Check sheet for the modelled part. Datum: model origin and axes. Units: mm. Face numbers are marked on the shaded views. A direction names the side the tool comes from. Coordinates: 2 decimals unless noted, no trailing zeros. Loops run counter-clockwise (first coordinate to the right, second up) from the corner with the lowest first, then second, coordinate; pieces in that order, holes last. Notation, with made-up numbers: M 71,42.5 L 109,42.5 A20 cw 109,62.5 Z; hole C 22.25,-23 d2. An arc over 180 degrees is marked long. Write each question's results on one line, items separated by ' | '. Start each with the question number.
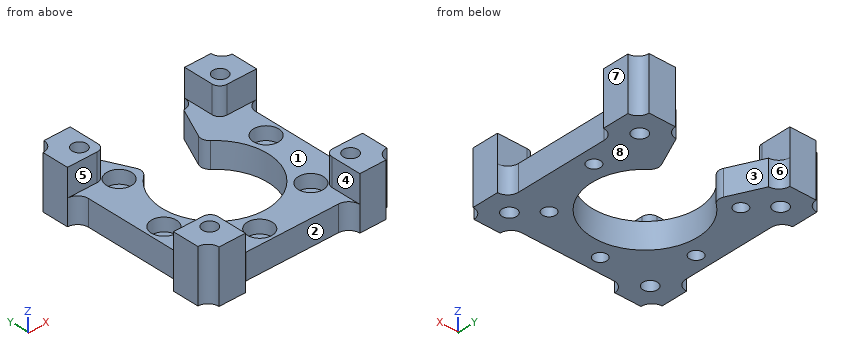
from build123d import *

# Parameters (mm, degrees)
SKETCH_R     = 1.5
SKETCH_R_2   = 1.65
PAD_DEPTH    = 5.8
SKETCH001_R  = 1.65
PAD001_DEPTH = 6.2
SKETCH002_R  = 2.85
POCKET_DEPTH = 3


with BuildPart() as part:
    # Sketch → Pad (new body)
    with BuildSketch(Plane.XY):
        with BuildLine():
            ThreePointArc((-21.5, 19), (-19.732233, 19.732233), (-19, 21.5))
            Line((-19, 21.5), (-13, 21.5))
            ThreePointArc((-13, 21.5), (-12.267767, 19.732233), (-10.500001, 19))
            Line((-10.500001, 19), (-7.065457, 11.675563))
            ThreePointArc((-7.608223, 9.279814), (-6.925691, 10.384542), (-7.065457, 11.675563))
            ThreePointArc((-7.608223, 9.279814), (0, -12), (7.608223, 9.279814))
            ThreePointArc((7.065457, 11.675563), (6.925691, 10.384541), (7.608223, 9.279814))
            Line((10.500001, 19), (7.065457, 11.675563))
            ThreePointArc((10.500001, 19), (12.267767, 19.732233), (13, 21.5))
            Line((19, 21.5), (13, 21.5))
            ThreePointArc((19, 21.5), (19.732233, 19.732233), (21.5, 19))
            Line((21.5, 19), (21.5, 13))
            ThreePointArc((21.5, 13), (19.732233, 12.267767), (19, 10.500001))
            Line((19, 10.500001), (19, -10.500001))
            ThreePointArc((19, -10.500001), (19.732233, -12.267767), (21.5, -13))
            Line((21.5, -19), (21.5, -13))
            ThreePointArc((21.5, -19), (19.732233, -19.732233), (19, -21.5))
            Line((19, -21.5), (13, -21.5))
            ThreePointArc((13, -21.5), (12.267767, -19.732233), (10.500001, -19))
            Line((10.500001, -19), (-10.500001, -19))
            ThreePointArc((-10.500001, -19), (-12.267767, -19.732233), (-13, -21.5))
            Line((-19, -21.5), (-13, -21.5))
            ThreePointArc((-19, -21.5), (-19.732233, -19.732233), (-21.5, -19))
            Line((-21.5, -19), (-21.5, -13))
            ThreePointArc((-21.5, -13), (-19.732233, -12.267767), (-19, -10.500001))
            Line((-19, 10.500001), (-19, -10.500001))
            ThreePointArc((-19, 10.500001), (-19.732233, 12.267767), (-21.5, 13))
            Line((-21.5, 19), (-21.5, 13))
        make_face()
        with Locations((-11.313708, 11.313708)):
            Circle(SKETCH_R, mode=Mode.SUBTRACT)
        with Locations((-15.454813, -4.141105)):
            Circle(SKETCH_R, mode=Mode.SUBTRACT)
        with Locations((-4.141105, -15.454813)):
            Circle(SKETCH_R, mode=Mode.SUBTRACT)
        with Locations((11.313708, -11.313708)):
            Circle(SKETCH_R, mode=Mode.SUBTRACT)
        with Locations((15.454813, 4.141105)):
            Circle(SKETCH_R, mode=Mode.SUBTRACT)
        with Locations((-16, 16)):
            Circle(SKETCH_R_2, mode=Mode.SUBTRACT)
        with Locations((16, 16)):
            Circle(SKETCH_R_2, mode=Mode.SUBTRACT)
        with Locations((16, -16)):
            Circle(SKETCH_R_2, mode=Mode.SUBTRACT)
        with Locations((-16, -16)):
            Circle(SKETCH_R_2, mode=Mode.SUBTRACT)
    extrude(amount=PAD_DEPTH)

    # Sketch001 (on Face39 of Pad) → Pad001 (join)
    with BuildSketch(Plane.XY.offset(5.8)):
        with BuildLine():
            ThreePointArc((-21.5, 19), (-19.732233, 19.732233), (-19, 21.5))
            Line((-19, 21.5), (-13, 21.5))
            Line((-13, 21.5), (-13, 14.726703))
            ThreePointArc((-14.726703, 13), (-13.50574, 13.50574), (-13, 14.726703))
            Line((-21.5, 13), (-14.726703, 13))
            Line((-21.5, 19), (-21.5, 13))
        make_face()
        with Locations((-16, 16)):
            Circle(SKETCH001_R, mode=Mode.SUBTRACT)
        with BuildLine():
            ThreePointArc((-19, -21.5), (-19.732233, -19.732233), (-21.5, -19))
            Line((-21.5, -19), (-21.5, -13))
            Line((-21.5, -13), (-14.726703, -13))
            ThreePointArc((-13, -14.726703), (-13.50574, -13.50574), (-14.726703, -13))
            Line((-13, -21.5), (-13, -14.726703))
            Line((-19, -21.5), (-13, -21.5))
        make_face()
        with Locations((-16, -16)):
            Circle(SKETCH001_R, mode=Mode.SUBTRACT)
        with BuildLine():
            ThreePointArc((21.5, -19), (19.732233, -19.732233), (19, -21.5))
            Line((19, -21.5), (13, -21.5))
            Line((13, -21.5), (13, -14.726703))
            ThreePointArc((14.726703, -13), (13.50574, -13.50574), (13, -14.726703))
            Line((21.5, -13), (14.726703, -13))
            Line((21.5, -19), (21.5, -13))
        make_face()
        with Locations((16, -16)):
            Circle(SKETCH001_R, mode=Mode.SUBTRACT)
        with BuildLine():
            ThreePointArc((19, 21.5), (19.732233, 19.732233), (21.5, 19))
            Line((21.5, 19), (21.5, 13))
            Line((21.5, 13), (14.726703, 13))
            ThreePointArc((13, 14.726703), (13.50574, 13.50574), (14.726703, 13))
            Line((13, 21.5), (13, 14.726703))
            Line((19, 21.5), (13, 21.5))
        make_face()
        with Locations((16, 16)):
            Circle(SKETCH001_R, mode=Mode.SUBTRACT)
    extrude(amount=PAD001_DEPTH)

    # Sketch002 (on Face4 of Pad001) → Pocket (cut)
    with BuildSketch(Plane.XY.offset(5.8)):
        with Locations((-11.313708, 11.313708)):
            Circle(SKETCH002_R)
        with Locations((15.454813, 4.141105)):
            Circle(SKETCH002_R)
        with Locations((11.313708, -11.313708)):
            Circle(SKETCH002_R)
        with Locations((-4.141105, -15.454813)):
            Circle(SKETCH002_R)
        with Locations((-15.454813, -4.141105)):
            Circle(SKETCH002_R)
    extrude(amount=-POCKET_DEPTH, mode=Mode.SUBTRACT)


solid = part.part
1) Section check B-B (y = 0). Enter the section's corners in (x, z), then the cut area to 3 significant figures.
2) Release check for a two-part mould opening along X. For the marked faces 6, 7 and 8 record: +X half, -X half, draft (parallel to the pull), parting line (faces both ways), or undercut.
3) Section check A-A (z = 7.25). Enter the section's corners in (x, y), then the cut area to 3 significant figures.
4) Gauge pin test, flat ends, axial feed: P1, Ø1.7, axis at x = 1, z = 3, coming from the -Y side; P2, Ø2, axis at y = -10.5, z = 3.5, coming from the +X side; P3, Ø6, axis at y = 6.5, z = 3.5, coming from the +X side. Record the tip position at first contact, or that the pin passes through.
5) Thickness scan on probe 1 along Y at (x, z) = (16, 6); probe 2 along X at (y, z) = (4.5, 2); probe 3 along Y at (x, z) = (-15, 7). Record the ranges inside material, lowest first.
6) Section check C-C (y = 16). Enter the section's corners in (x, z), then the cut area to 3 significant figures.
7) Section check D-D (x = -2). Enter the section's corners in (y, z).
8) Set-up check for the marked faces 1, 2, 3, 4 and 5: record each of +Z, -Z, +X, -X, +Y, -Y from which the full face is reachable in a straight line by a thin tool's end or side.
Return value:
1) outline: M -19,0 L -12,0 L -12,5.8 L -19,5.8 Z; M 12,0 L 19,0 L 19,5.8 L 12,5.8 Z | area: 81.2 mm2
2) face 6: undercut | face 7: +X half | face 8: draft
3) outline: M -21.5,-19 A2.5 cw -19,-21.5 L -13,-21.5 L -13,-14.73 A1.73 ccw -14.73,-13 L -21.5,-13 Z; M -21.5,13 L -14.73,13 A1.73 ccw -13,14.73 L -13,21.5 L -19,21.5 A2.5 cw -21.5,19 Z; M 13,-21.5 L 19,-21.5 A2.5 cw 21.5,-19 L 21.5,-13 L 14.73,-13 A1.73 ccw 13,-14.73 Z; M 13,14.73 A1.73 ccw 14.73,13 L 21.5,13 L 21.5,19 A2.5 cw 19,21.5 L 13,21.5 Z; hole C -16,-16 d3.3; hole C -16,16 d3.3; hole C 16,-16 d3.3; hole C 16,16 d3.3 | area: 233 mm2
4) P1: stops at y = -19 | P2: stops at x = 19.21 | P3: stops at x = 19
5) probe 1: y = -21.5 to -17.65, -14.35 to -13, 13 to 14.35, 17.65 to 21.5 | probe 2: x = -19 to -11.12, 11.12 to 14, 16.91 to 19 | probe 3: y = -21.5 to -17.31, -14.69 to -13, 13 to 14.69, 17.31 to 21.5
6) outline: M -21.5,0 L -17.65,0 L -17.65,12 L -21.5,12 Z; M -14.35,0 L -9.09,0 L -9.09,5.8 L -13,5.8 L -13,12 L -14.35,12 Z; M 9.09,0 L 14.35,0 L 14.35,12 L 13,12 L 13,5.8 L 9.09,5.8 Z; M 17.65,0 L 21.5,0 L 21.5,12 L 17.65,12 Z | area: 170 mm2
7) outline: M -19,0 L -11.83,0 L -11.83,5.8 L -13.57,5.8 L -13.57,2.8 L -17.34,2.8 L -17.34,5.8 L -19,5.8 Z
8) face 1: +Z | face 2: +Z, -Z, -Y | face 3: +Z, -Z, +Y | face 4: +Z, +Y, -Y | face 5: +Z, +X, -X
